The drawing under review shows one solid part. Ordinate dimensions are in mm from its lowest x, y, z. A direction names the side the tool comes from. Give positions to 0.01 mm unless a question says otherwise; leave off trailing zeros. Loops run counter-clockwise (first coordinate to the right, second up) from the corner with the lowest first, then second, coordinate; pieces in that order, holes last. Notation, with made-up numbers: M 67.25,-23.5 L 95.25,-23.5 A32 ccw 95.25,15.5 Z; hole C 4,0.5 d10. An arc over 180 degrees is marked long. One line per item, written item: value. Start each with the question number.
Q1. We need section B-B on z = 3.25. Write out the cut boundary in (x, y).
Q2. To check wall thickness, follow line 1 along Y through (x, z) = (5.75, 1.5); line 2 along Z through (x, y) = (2.75, 14.25); line 3 along Z through (x, y) = (3, 14). State the ranges of each line that lie inside material, in increasing order. Write a range as from..to.
Q3. We need section D-D on y = 1.25. Write out the cut boundary in (x, z), plus the area to 3 significant figures.
Q4. We need section C-C on y = 16. Write out the cut boundary in (x, z).
Q5. For the marked faces 1 and 2, list the 3-axis set-ups (+Z, -Z, +X, -X, +Y, -Y) from which the entire face can be reached by the end or side of a thin tool; tool diameter is ignored.
Q6. For pin 1 (3 mm diameter, centred on x = 2, y = 13, fed in from -Z); pin 2 (1.5 mm diameter, centred on x = 5, y = 8.5, fed in from +Z), all flat-tipped, find the tip position at first contact; note any pin that passes through.
Q7. We need section A-A on x = 3.25. Write out the cut boundary in (y, z).
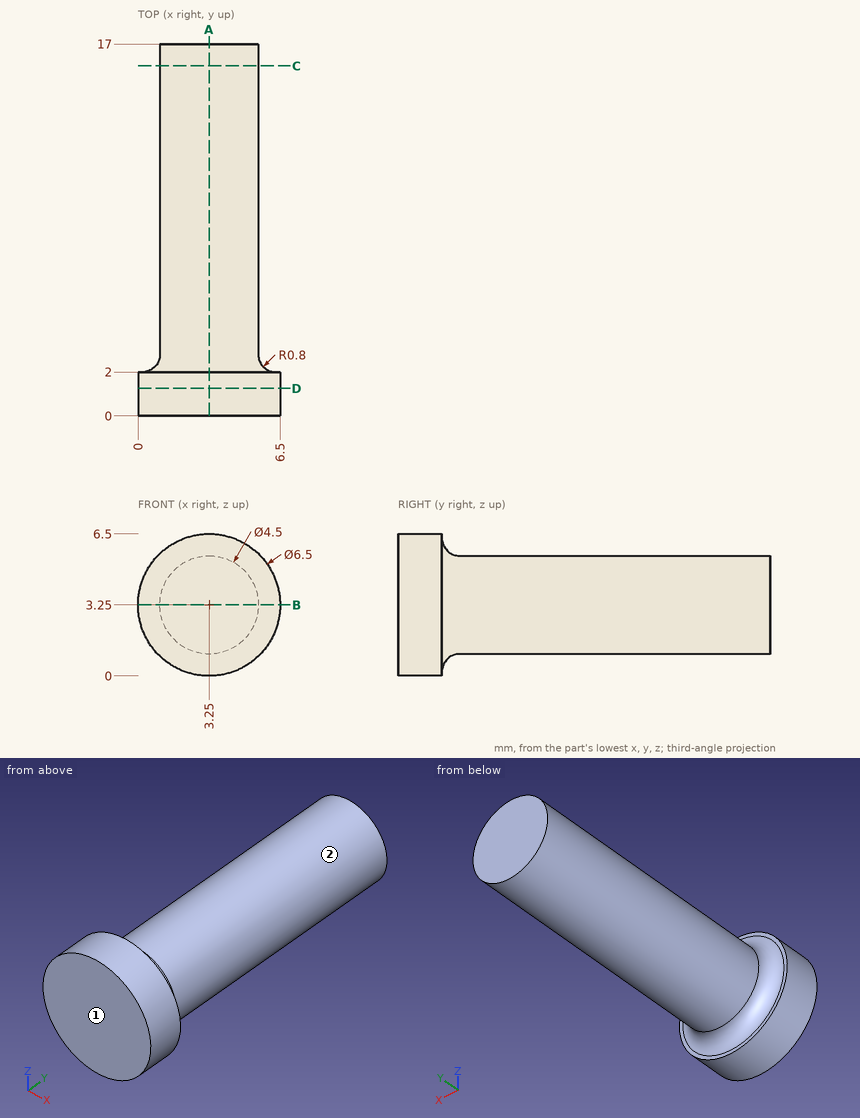
Solved:
1. outline: M 0,0 L 6.5,0 L 6.5,2 L 6.3,2 A0.8 cw 5.5,2.8 L 5.5,17 L 1,17 L 1,2.8 A0.8 cw 0.2,2 L 0,2 Z
2. line 1: 0..2
2. line 2: 1.06..5.44
2. line 3: 1.01..5.49
3. outline: C 3.25,3.25 d6.5
3. area: 33.2 mm2
4. outline: C 3.25,3.25 d4.5
5. face 1: +Z, -Z, +X, -X, -Y
5. face 2: +Y
6. pin 1: z = 1
6. pin 2: z = 5.27
7. outline: M 0,0 L 2,0 L 2,0.2 A0.8 cw 2.8,1 L 17,1 L 17,5.5 L 2.8,5.5 A0.8 cw 2,6.3 L 2,6.5 L 0,6.5 Z
